```python
from build123d import *

# Parameters (mm, degrees)
SKETCH1_R           = 3
SKETCH1_W           = 2
SKETCH1_H           = 1.17
BOSS_EXTRUDE1_DEPTH = 27.5
SKETCH2_R           = 6.166150273
SKETCH2_R_2         = 1.95
CUT_EXTRUDE1_DEPTH  = 22
CUT_EXTRUDE2_DEPTH  = 7
CUT_EXTRUDE3_DEPTH  = 100


with BuildPart() as part:
    # Sketch1 → Boss-Extrude1 (new body)
    with BuildSketch(Plane(origin=(0, 0, 0), x_dir=(1, 0, 0), z_dir=(0, 1, 0))):
        Circle(SKETCH1_R)
        with Locations((0, 3.413427125)):
            Rectangle(SKETCH1_W, SKETCH1_H)
    extrude(amount=BOSS_EXTRUDE1_DEPTH)

    # Sketch2 → Cut-Extrude1 (cut)
    with BuildSketch(Plane(origin=(0, 27.5, 0), x_dir=(1, 0, 0), z_dir=(0, 1, 0))):
        Circle(SKETCH2_R)
        Circle(SKETCH2_R_2, mode=Mode.SUBTRACT)
    extrude(amount=-CUT_EXTRUDE1_DEPTH, mode=Mode.SUBTRACT)

    # Sketch3 → Cut-Extrude2 (cut)
    with BuildSketch(Plane(origin=(0, 27.5, 0), x_dir=(1, 0, 0), z_dir=(0, 1, 0))):
        with BuildLine():
            Line((-0.975, 1.688749537), (-0.975, -1.688749537))
            ThreePointArc((-0.975, -1.688749537), (-1.95, 0), (-0.975, 1.688749537))
        make_face()
        with BuildLine():
            Line((0.975, 1.688749537), (0.975, -1.688749537))
            ThreePointArc((0.975, -1.688749537), (1.95, 0), (0.975, 1.688749537))
        make_face()
    extrude(amount=-CUT_EXTRUDE2_DEPTH, mode=Mode.SUBTRACT)

    # Sketch4 → Cut-Extrude3 (cut)
    with BuildSketch(Plane.XZ):
        with BuildLine():
            Line((-1, -3.998427125), (1, -3.998427125))
            Line((1, -3.998427125), (1, -2.828427125))
            ThreePointArc((1, -2.828427125), (0, 3), (-1, -2.828427125))
            Line((-1, -2.828427125), (-1, -3.998427125))
        make_face()
        with BuildLine():
            Line((-0.9, -2.75680975), (-0.9, -3.898427125))
            Line((-0.9, -3.898427125), (0.9, -3.898427125))
            Line((0.9, -3.898427125), (0.9, -2.75680975))
            ThreePointArc((0.9, -2.75680975), (0, 2.9), (-0.9, -2.75680975))
        make_face(mode=Mode.SUBTRACT)
    extrude(amount=-CUT_EXTRUDE3_DEPTH, mode=Mode.SUBTRACT)


solid = part.part
```
Input: part model. Units: mm. Frame: model coordinates. A direction names the side the tool comes from. Coordinates: 2 decimals unless noted, no trailing zeros. Loops run counter-clockwise (first coordinate to the right, second up) from the corner with the lowest first, then second, coordinate; pieces in that order, holes last. Notation, with made-up numbers: (-13, 14) - (13, 14) arc R4 ccw to (13, 18) - close; hole circle Ø10 at (-13, -16.75). An arc over 180 degrees is marked (long way). Answer in a Markdown table with one row per item.
(1) Cut plane D-D on y = 4. Output: boundary loops of the cut face in (x, z).
Model answer:
| item | result |
|---|---|
| outline | (-0.9, -3.9) - (0.9, -3.9) - (0.9, -2.76) arc R2.9 ccw (long way) to (-0.9, -2.76) - close |
(2) Material intervals for L1, parallel to Y at x = -1.2, z = -0.5; L2, parallel to X at y = 25.5, z = -0.75 (3 decimals); L3, parallel to Z at x = 0.1, y = 17, sorted ascending. Write a range as from..to.
Model answer:
| item | result |
|---|---|
| L1 | y = 0..20.5 |
| L2 | x = -0.975..0.975 |
| L3 | z = -1.95..1.95 |
(3) Pin query (flat end, axial travel): P1, Ø1, axis at x = 1.5, y = 7.5, coming from the -Z side; P2, Ø0.6, axis at y = 4, z = -3.5, coming from the +X side; P3, Ø0.8, axis at x = 1.5, z = 0, coming from the +Y side. Return the tip coordinate at first contact, or that it passes through.
Model answer:
| item | result |
|---|---|
| P1 | stops at z = -1.67 |
| P2 | stops at x = 0.9 |
| P3 | stops at y = 20.5 |
(4) Cut plane B-B on x = 0. Output: boundary loops of the cut face in (y, z).
Model answer:
| item | result |
|---|---|
| outline | (0, -3.9) - (5.5, -3.9) - (5.5, -1.95) - (27.5, -1.95) - (27.5, 1.95) - (5.5, 1.95) - (5.5, 2.9) - (0, 2.9) - close |
(5) Cut plane A-A on z = 0. Output: boundary loops of the cut face in (x, y) (3 decimals), plus the area to 3 significant figures.
Model answer:
| item | result |
|---|---|
| outline | (-2.9, 0) - (2.9, 0) - (2.9, 5.5) - (1.95, 5.5) - (1.95, 20.5) - (0.975, 20.5) - (0.975, 27.5) - (-0.975, 27.5) - (-0.975, 20.5) - (-1.95, 20.5) - (-1.95, 5.5) - (-2.9, 5.5) - close |
| area | 104 mm² |
(6) Cut plane C-C on y = 25.5. Output: boundary loops of the cut face in (x, z) (3 decimals).
Model answer:
| item | result |
|---|---|
| outline | (-0.975, -1.689) arc R1.95 ccw to (0.975, -1.689) - (0.975, 1.689) arc R1.95 ccw to (-0.975, 1.689) - close |
(7) Set-up query: faces 1 (the face through (-0.9, 3, -3)), 2 (the face through (0.9, 3, -3)), 3 (the face through (1.3, 20.5, 0)). Return all of +Z, -Z, +X, -X, +Y, -Y with unobstructed straight access to the full face (end or side cutting, diameter ignored); none if empty.
Model answer:
| item | result |
|---|---|
| face 1 | -Z, -X, +Y, -Y |
| face 2 | -Z, +X, +Y, -Y |
| face 3 | +Z, -Z, +X, +Y |
